Autodesk Inventor part; units mm, degrees
ref_plane "YZ Plane" through (0, 0, 0) normal (1, 0, 0) x (0, 1, 0)
ref_plane "XZ Plane" through (0, 0, 0) normal (0, 1, 0) x (-1, 0, 0)
ref_plane "XY Plane" through (0, 0, 0) normal (0, 0, 1) x (1, 0, 0)
sketch "Sketch1" plane through (0, 0, 0) normal (1, 0, 0) x (0, 1, 0)
  line L0 (1.5, -2) -> (-1.5, -2)
  line L1 (1.5, -2) -> (1.5, -4)
  line L2 (1.5, -4) -> (1.2, -4.5)
  line L3 (1.2, -4.5) -> (1.5, -5)
  line L4 (1.5, -5) -> (3.1, -5)
  line L5 (3.1, -5) -> (3.1, 0)
  line L6 (3.1, 0) -> (-3.1, 0)
  line L7 (-3.1, 0) -> (-3.1, -5)
  line L8 (-3.1, -5) -> (-1.5, -5)
  line L9 (-1.5, -5) -> (-1.2, -4.5)
  line L10 (-1.2, -4.5) -> (-1.5, -4)
  line L11 (-1.5, -4) -> (-1.5, -2)
  point P0 (0, 0)
  point P1 (0, -2)
  dimension "d0" = 3
  dimension "d1" = 2
  dimension "d2" = 1.6
  dimension "d3" = 1.6
  dimension "d4" = 0.3
  dimension "d5" = 3
  dimension "d6" = 2
extrude "Extrusion1" add sketch "Sketch1" along normal blind 50
fillet "Fillet1" radius 2 2 edges at (25, 3.1, 0) (25, -3.1, 0)
properties part number "ForceStopper" material "ABS Plastic"
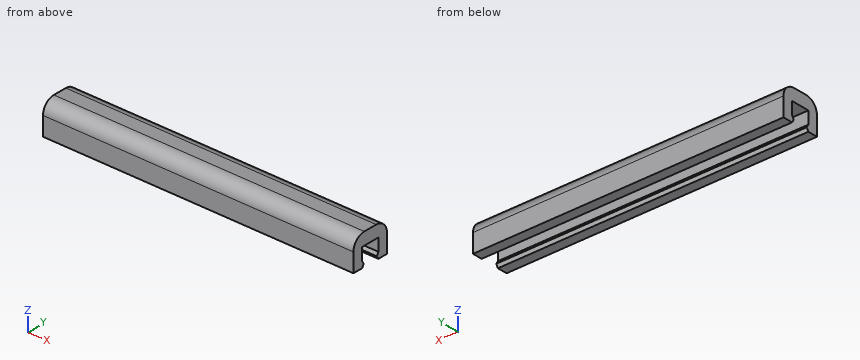
Work out the finished part from the listing and answer in its coordinate system (mm). Coordinates: 2 decimals unless noted, no trailing zeros. Loops run counter-clockwise (first coordinate to the right, second up) from the corner with the lowest first, then second, coordinate; pieces in that order, holes last. Notation, with made-up numbers: (10, -33) -> (66, -33) arc R34 cw to (66, 3) -> close; hole circle Ø1 at (54, 41). An arc over 180 degrees is marked (long way). Write each question's results on one line, items separated by ' | '. Start each with the question number.
1) Find section C-C on y = -0.5. Determine the outline of the cut face in (x, z), then the cut area to 3 significant figures.
2) Find section D-D on z = -1.4. Determine the outline of the cut face in (x, y), then the cut area to 3 significant figures.
3) Consider line 1 along Y through (x, z) = (27, -2.55); line 2 along Z through (x, y) = (23, 0.5); line 3 along Y through (x, z) = (19.5, -1.85). Determine where each line is inside the solid, lowest interval first.
4) Find section A-A on z = -3.5. Determine the outline of the cut face in (x, y), then the cut area to 3 significant figures.
5) A flat-ended cylindrical pin translates along its axis: P1, Ø1.5, axis at x = 28.5, y = 0, coming from the -Z side. Find the tip coordinate at first contact, or state that the pin passes through.
6) Find section B-B on x = 11.5. Determine the outline of the cut face in (y, z), then the cut area to 3 significant figures.
Response values:
1) outline: (0, -2) -> (50, -2) -> (50, 0) -> (0, 0) -> close | area: 100 mm^2
2) outline: (0, -3.01) -> (50, -3.01) -> (50, 3.01) -> (0, 3.01) -> close | area: 301 mm^2
3) line 1: y = -3.1 to -1.5, 1.5 to 3.1 | line 2: z = -2 to 0 | line 3: y = -3.09 to 3.09
4) outline: (0, -3.1) -> (50, -3.1) -> (50, -1.5) -> (0, -1.5) -> close; (0, 1.5) -> (50, 1.5) -> (50, 3.1) -> (0, 3.1) -> close | area: 160 mm^2
5) P1: stops at z = -2
6) outline: (-3.1, -5) -> (-1.5, -5) -> (-1.2, -4.5) -> (-1.5, -4) -> (-1.5, -2) -> (1.5, -2) -> (1.5, -4) -> (1.2, -4.5) -> (1.5, -5) -> (3.1, -5) -> (3.1, -2) arc R2 ccw to (1.1, 0) -> (-1.1, 0) arc R2 ccw to (-3.1, -2) -> close | area: 20.6 mm^2
